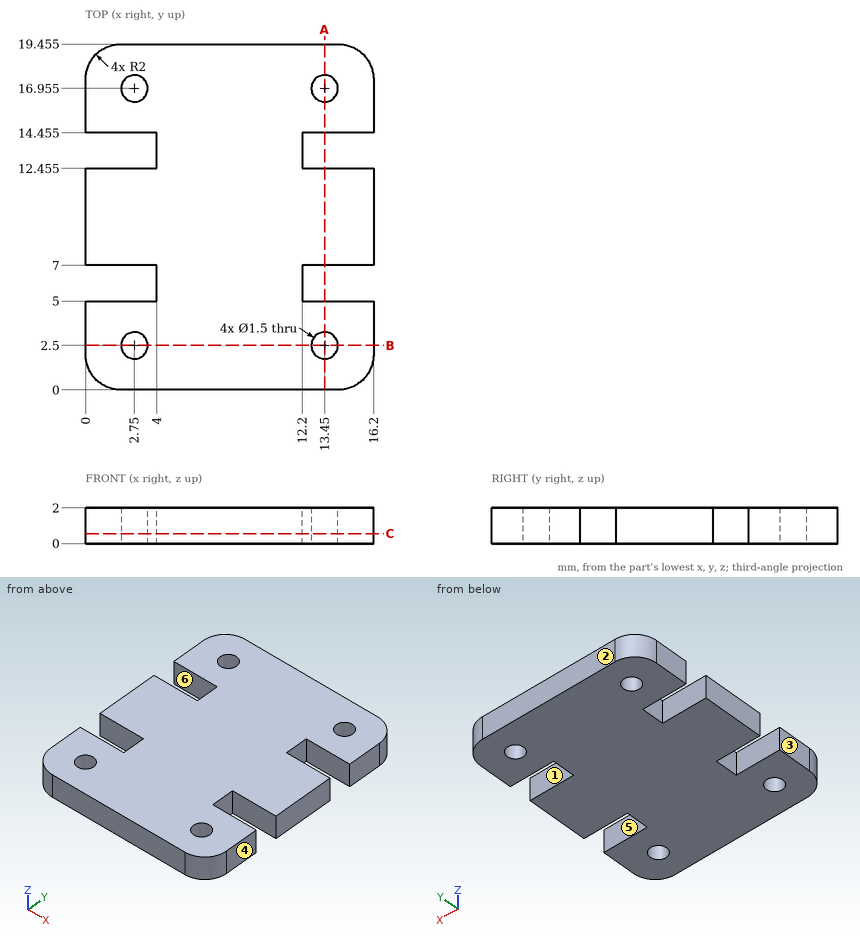
Geometry check sheet. Reference: drawing and pictorial views, mm from the part's lowest x, y, z. A direction names the side the tool comes from. Round coordinates to 2 decimals unless told otherwise and drop trailing zeros. Write each loop counter-clockwise with the first axis right and the second up, starting at its lowest first coordinate (ties: lowest second). Pieces come first, ordered by that corner, then holes. Notation, with made-up numbers: (59, 36) -> (110, 36) arc R24 ccw to (110, 61) -> close; hole circle Ø11 at (-36, 82.5). An arc over 180 degrees is marked (long way). Put each result on its own line as item: value.
1) Thickness scan on probe 1 along Y at (x, z) = (2.75, 1.35) (3 decimals); probe 2 along Y at (x, z) = (15.25, 0.15) (3 decimals); probe 3 along Y at (x, z) = (13.75, 0.5) (3 decimals). Record the ranges inside material, lowest first. Write a range as from..to.
Recorded:
probe 1: y = 0..1.75, 3.25..5, 7..12.455, 14.455..16.205, 17.705..19.455
probe 2: y = 0.298..5, 7..12.455, 14.455..19.157
probe 3: y = 0..1.813, 3.187..5, 7..12.455, 14.455..16.268, 17.642..19.455
2) Release check for a two-part mould opening along Y. For the marked faces 1, 2 and 3 record: pulls with the +Y half, pulls with the -Y half, needs draft (parallel to the pull), parting line crosses it, or undercut.
Recorded:
face 1: undercut
face 2: pulls with the +Y half
face 3: needs draft
3) Cross-section at C-C, the plane z = 0.55. Enter the section's corners in (x, y) (3 decimals), plus the area to 3 significant figures.
Recorded:
outline: (0, 2) arc R2 ccw to (2, 0) -> (14.2, 0) arc R2 ccw to (16.2, 2) -> (16.2, 5) -> (12.2, 5) -> (12.2, 7) -> (16.2, 7) -> (16.2, 12.455) -> (12.2, 12.455) -> (12.2, 14.455) -> (16.2, 14.455) -> (16.2, 17.455) arc R2 ccw to (14.2, 19.455) -> (2, 19.455) arc R2 ccw to (0, 17.455) -> (0, 14.455) -> (4, 14.455) -> (4, 12.455) -> (0, 12.455) -> (0, 7) -> (4, 7) -> (4, 5) -> (0, 5) -> close; hole circle Ø1.5 at (2.75, 2.5); hole circle Ø1.5 at (2.75, 16.955); hole circle Ø1.5 at (13.45, 2.5); hole circle Ø1.5 at (13.45, 16.955)
area: 273 mm2
4) Cross-section at A-A, the plane x = 13.45. Enter the section's corners in (y, z) (3 decimals), plus the area to 3 significant figures.
Recorded:
outline: (0, 0) -> (1.75, 0) -> (1.75, 2) -> (0, 2) -> close; (3.25, 0) -> (5, 0) -> (5, 2) -> (3.25, 2) -> close; (7, 0) -> (12.455, 0) -> (12.455, 2) -> (7, 2) -> close; (14.455, 0) -> (16.205, 0) -> (16.205, 2) -> (14.455, 2) -> close; (17.705, 0) -> (19.455, 0) -> (19.455, 2) -> (17.705, 2) -> close
area: 24.9 mm2
5) Access from +Z, -Z, +X, -X, +Y, -Y to the whole of each face (thin tool, end or side, straight path). Record for the marked faces 4, 5 and 6.
Recorded:
face 4: +Z, -Z, +X, +Y, -Y
face 5: +Z, -Z, +X
face 6: +Z, -Z, -X
6) Depth check by flat-ended pin: P1, Ø1, axis at y = 6, z = 1.5, coming from the -X side. Enter the tip coordinate at first touch or a pass-through.
Recorded:
P1: stops at x = 4
7) Cross-section at B-B, the plane y = 2.5. Enter the section's corners in (x, z).
Recorded:
outline: (0, 0) -> (2, 0) -> (2, 2) -> (0, 2) -> close; (3.5, 0) -> (12.7, 0) -> (12.7, 2) -> (3.5, 2) -> close; (14.2, 0) -> (16.2, 0) -> (16.2, 2) -> (14.2, 2) -> close
